from build123d import *

# Parameters (mm, degrees)
SKETCH1_W                  = 50.8
SKETCH1_H                  = 25.4
BASE_DEPTH                 = 101.6
SKETCH2_R                  = 10.999999971
LEADNUT_FLANGE_INSET_DEPTH = 4.999999906
SKETCH3_R                  = 5.09999996
LEADNUT_THROUGH_HOLE_DEPTH = 113.059627066
LEADNUT_HOLE_PATTERN_D     = 2.9
LEADNUT_HOLE_PATTERN_DEPTH = 10.0000054
LEADNUT_HOLE_PATTERN_TIP   = 0.871247898


with BuildPart() as part:
    # Sketch1 → base (new body)
    with BuildSketch(Plane.XY):
        with Locations((25.4, 12.7)):
            Rectangle(SKETCH1_W, SKETCH1_H)
    extrude(amount=BASE_DEPTH)

    # Sketch2 → leadnut_flange_inset (cut)
    with BuildSketch(Plane.XY.offset(101.6)):
        with Locations((25.4, 12.7)):
            Circle(SKETCH2_R)
    extrude(amount=-LEADNUT_FLANGE_INSET_DEPTH, mode=Mode.SUBTRACT)

    # Sketch3 → leadnut_through_hole (cut, through all)
    with BuildSketch(Plane.XY.offset(96.600000094)):
        with Locations((25.4, 12.7)):
            Circle(SKETCH3_R)
    extrude(amount=-LEADNUT_THROUGH_HOLE_DEPTH, mode=Mode.SUBTRACT)

    # leadnut_hole_pattern
    with Locations(Plane.XY.offset(96.600000094)):
        with Locations((25.4, 12.7), (25.4, 20.6999967), (17.4000033, 12.7), (25.4, 4.7000033), (33.3999967, 12.7)):
            Hole(LEADNUT_HOLE_PATTERN_D / 2, depth=LEADNUT_HOLE_PATTERN_DEPTH)
            with Locations((0, 0, -(LEADNUT_HOLE_PATTERN_DEPTH + LEADNUT_HOLE_PATTERN_TIP / 2))):  # 118° drill point
                Cone(0, LEADNUT_HOLE_PATTERN_D / 2, LEADNUT_HOLE_PATTERN_TIP, mode=Mode.SUBTRACT)


solid = part.part
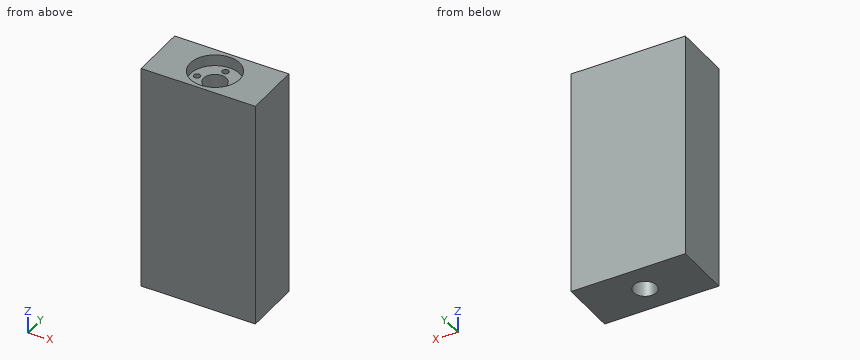
Here's how the part is built. I have some questions about the finished solid (model axes, mm). Coordinates: 2 decimals unless noted, no trailing zeros. Write each loop counter-clockwise with the first axis right and the second up, starting at its lowest first coordinate (ties: lowest second). Pieces come first, ordered by that corner, then holes. Notation, with made-up numbers: (82.25, 31.5) - (107.25, 31.5) arc R32 cw to (107.25, 60.5) - close; hole circle Ø9 at (-12, -24). An arc over 180 degrees is marked (long way). Use one line per item in the form item = value.
1) Suppose I cut it at B-B, the plane z = 75. Write out the boundary of the cut face in (x, y).
Solved:
outline = (0, 0) - (50.8, 0) - (50.8, 25.4) - (0, 25.4) - close; hole circle Ø10.2 at (25.4, 12.7)
2) I need wall thicknesses on line 1 (Y direction, x = 25, z = 89); line 2 (Y direction, x = 25.4, z = 38); line 3 (Z direction, x = 33.5, y = 9.25). Which ranges of each line are inside material? Lowest first, please.
Solved:
line_1 = 0 to 3.31, 6.09 to 7.62, 17.78 to 19.31, 22.09 to 25.4
line_2 = 0 to 7.6, 17.8 to 25.4
line_3 = 0 to 96.6
3) Suppose I cut it at A-A, the plane y = 16.75. Write out the boundary of the cut face in (x, z), plus the area to 3 significant figures.
Solved:
outline = (0, 0) - (22.3, 0) - (22.3, 96.6) - (15.17, 96.6) - (15.17, 101.6) - (0, 101.6) - close; (28.5, 0) - (50.8, 0) - (50.8, 101.6) - (35.63, 101.6) - (35.63, 96.6) - (28.5, 96.6) - close
area = 4,460 mm2
4) I'm going to push flat-ended pins straight in: P1, Ø1.5, axis at y = 13.5, z = 36, coming from the -X side; P2, Ø4.5, axis at x = 25.4, y = 20.7, coming from the +Z side; P3, Ø6, axis at x = 25.4, y = 12.7, coming from the -Z side; P4, Ø1.7, axis at x = 17.4, y = 12.7, coming from the +Z side. Where does each tip first touch, or does it pass through?
Solved:
P1 = 0
P2 = 96.6
P3 = through
P4 = 86.24
